from build123d import *
from build123d import SkipClean  # not in build123d's __all__

# Parameters (mm, degrees)
F0_R     = 4
F1_DEPTH = 3
F3_DEPTH = 25


# Not quite as in the source:
# - a feature names something its author has since deleted; it is built from what else it names


with BuildPart() as f1:
    # F0 (on Front) → F1 (new body)
    with BuildSketch(Plane.XZ):
        with BuildLine():
            Line((47.076298262, 17.7403006666), (-34.5741482174, 34.3593566285))
            ThreePointArc((-34.5741482174, 34.3593566285), (-40.7303881594, 32.6323986455), (-42.9151879903, 26.6233784428))
            ThreePointArc((-42.9151879903, 26.6233784428), (-39.7469745445, -1.0840101596), (-56.5827821886, -23.3167009679))
            ThreePointArc((-56.5827821886, -23.3167009679), (-56.7807033092, -31.4037364957), (-49.2188462892, -34.2773465607))
            Line((-49.2188462892, -34.2773465607), (47.076298262, -17.7403006666))
            ThreePointArc((47.076298262, -17.7403006666), (62.0297047119, 0), (47.076298262, 17.7403006666))
        make_face()
        with Locations((-50.9702952881, -27.5)):
            Circle(F0_R, mode=Mode.SUBTRACT)
        with Locations((-10.9702952881, 0)):
            Circle(F0_R, mode=Mode.SUBTRACT)
        with Locations((-35.9702952881, 27.5)):
            Circle(F0_R, mode=Mode.SUBTRACT)
        with Locations((14.0297047119, 0)):
            Circle(F0_R, mode=Mode.SUBTRACT)
        with BuildLine():
            ThreePointArc((36.818602161, -12), (30.0297047119, 0), (36.818602161, 12))
            Line((36.818602161, 12), (51.2408072628, 12))
            ThreePointArc((51.2408072628, 12), (58.0297047119, 0), (51.2408072628, -12))
            Line((51.2408072628, -12), (36.818602161, -12))
        make_face(mode=Mode.SUBTRACT)
    extrude(amount=F1_DEPTH)

    # F2 (on face) → F3 (cut)
    with BuildSketch(Plane.XZ.offset(3)):
        with BuildLine():
            ThreePointArc((33.9762752, 14.9307921776), (40.2551488392, 17.5997934068), (47.076298262, 17.7403006666))
            Line((47.076298262, 17.7403006666), (-10.9702952881, 29.555050349))
            ThreePointArc((-10.9702952881, 29.555050349), (7.9384350476, 11.2875267012), (33.9762752, 14.9307921776))
        make_face()
        with BuildLine():
            ThreePointArc((47.076298262, -17.7403006666), (40.1280392566, -17.572051863), (33.7614970255, -14.7839071598))
            ThreePointArc((33.7614970255, -14.7839071598), (8.3202088026, -10.6027369585), (-10.9702952881, -27.7088113948))
            Line((-10.9702952881, -27.7088113948), (47.076298262, -17.7403006666))
        make_face()
        with BuildLine():
            ThreePointArc((-30.363862552, 11.08172749), (-30.8978419926, -0.5969747066), (-34.8691691907, -11.5926911146))
            ThreePointArc((-34.8691691907, -11.5926911146), (-33.2604899055, -17.0159881706), (-27.8371928496, -15.4073088854))
            ThreePointArc((-27.8371928496, -15.4073088854), (-23.0512344312, -2.1560609065), (-22.4077207465, 11.91827251))
            ThreePointArc((-22.4077207465, 11.91827251), (-26.8040641592, 15.4780709028), (-30.363862552, 11.08172749))
        make_face()
    with SkipClean():  # cleaning this boolean's faces spoils the solid; the shape is the same uncleaned
        extrude(amount=-F3_DEPTH, mode=Mode.SUBTRACT)


solid = f1.part
The model under review builds one solid part; all positions refer to its coordinate system, in mm. A direction names the side the tool comes from. Round coordinates to 2 decimals unless told otherwise and drop trailing zeros. Loops run counter-clockwise (first coordinate to the right, second up) from the corner with the lowest first, then second, coordinate; pieces in that order, holes last. Notation, with made-up numbers: M 59,74.25 L 92,74.25 A8 ccw 92,86.25 Z; hole C -36.75,-39 d1. An arc over 180 degrees is marked long. Answer as CSV lines item,"result". Start each with the question number.
Item 1: Consider section D-D (y = -2.25). Write out the cut boundary in (x, z), then the cut area to 3 significant figures.
Item 2: Consider section B-B (z = -7). Write out the cut boundary in (x, y), then the cut area to 3 significant figures.
Item 3: Consider section C-C (x = 14). Write out the cut boundary in (y, z).
Item 4: Insertion check: P1, Ø1.5, axis at x = 44.5, y = -2, coming from the +Z side; P2, Ø5, axis at x = -35.5, z = 2, coming from the +Y side; P3, Ø1.5, axis at x = 43, y = -1.5, coming from the -Z side; P4, Ø1.5, axis at x = 20.5, y = -0.5, coming from the -Z side. Each pin has a flat end and moves straight along its axis. Give the tip position at first contact, or say it passes through.
Item 5: For faces 1 (the face through (-23.1, -1.5, -2.4)), 2 (the face through (7.6, -1.5, 11.4)), list the 3-axis set-ups (+Z, -Z, +X, -X, +Y, -Y) from which the entire face can be reached by the end or side of a thin tool; tool diameter is ignored.
Item 6: Consider section A-A (z = 0). Write out the cut boundary in (x, y), then the cut area to 3 significant figures.
Item 7: Wall thickness on line 1 (X direction, y = -1.9, z = -8.5); line 2 (X direction, y = -1.7, z = -2); line 3 (X direction, y = -0.3, z = 12.5): over which ranges is each line inside the solid? List them lowest first. Write a range as [from, to].
Answer:
1,outline,"M -56.58,-23.32 A7 ccw -49.22,-34.28 L -10.97,-27.71 A30 cw 33.76,-14.78 A18 ccw long 33.98,14.93 A30 cw -10.97,29.56 L -34.57,34.36 A7 ccw -42.92,26.62 A37.5 cw Z; hole C -50.97,-27.5 d8; hole C -35.97,27.5 d8; hole M -34.87,-11.59 A4 ccw -27.84,-15.41 A47 ccw -22.41,11.92 A4 ccw -30.36,11.08 A39 cw Z; hole C -10.97,0 d8; hole C 14.03,0 d8; hole M 36.82,-12 L 51.24,-12 A14 ccw 51.24,12 L 36.82,12 A14 ccw Z"
1,area,"3,160 mm^2"
2,outline,"M -41.91,-3 L -32.75,-3 L -32.75,0 L -41.91,0 Z; M -24.28,-3 L 31.91,-3 L 31.91,0 L -24.28,0 Z; M 56.15,-3 L 60.61,-3 L 60.61,0 L 56.15,0 Z"
2,area,"209 mm^2"
3,outline,"M -3,-9.54 L 0,-9.54 L 0,-4 L -3,-4 Z; M -3,4 L 0,4 L 0,9.99 L -3,9.99 Z"
4,P1,"stops at z = 18"
4,P2,"stops at y = 0"
4,P3,"stops at z = -18"
4,P4,"stops at z = -9.78"
5,face 1,"+Y, -Y"
5,face 2,"+Z, +Y, -Y"
6,outline,"M -39.47,-3 L -30.78,-3 L -30.78,0 L -39.47,0 Z; M -22.67,-3 L -14.97,-3 L -14.97,0 L -22.67,0 Z; M -6.97,-3 L 10.03,-3 L 10.03,0 L -6.97,0 Z; M 18.03,-3 L 30.03,-3 L 30.03,0 L 18.03,0 Z; M 58.03,-3 L 62.03,-3 L 62.03,0 L 58.03,0 Z"
6,area,"148 mm^2"
7,line 1,"x = [-42.65, -33.36], [-24.78, 32.91], [55.15, 59.9]"
7,line 2,"x = [-40.01, -31.2], [-23.02, -14.43], [-7.51, 10.57], [17.49, 30.17], [57.89, 61.92]"
7,line 3,"x = [-38.6, -30.26], [-22.51, 4.82], [29.62, 56.98]"
